Model file for the job. Use its own axes, mm. Face numbers are marked on the shaded views. A direction names the side the tool comes from. Coordinates: 2 decimals unless noted, no trailing zeros. Write each loop counter-clockwise with the first axis right and the second up, starting at its lowest first coordinate (ties: lowest second). Pieces come first, ordered by that corner, then holes.
Q1. Which spindle directions (+Z, -Z, +X, -X, +Y, -Y) get a long thin tool onto all of the face, cutting with end or side? Do the marked faces 1 and 2. Say none if no direction does.
Q2. Band-saw the part on A-A, the plane x = 0. State how many separate pieces and enclosed holes the cut face has, plus the area to 3 significant figures.
Q3. Band-saw the part on B-B, the plane y = -3.4. Write the cut outline in (x, z), plus the area to 3 significant figures.
Q4. Pull direction Z, two halves, no side cores. Call the marked faces 3, 4, 5 and 6: released by +Z, released by -Z, zero draft, split by the parting line, or undercut.
Q5. Pin check, flat tips, straight feed: P1, Ø1.5, axis at y = -4, z = 4, coming from the -X side; P2, Ø2, axis at y = -2, z = -3, coming from the +X side; P3, Ø1, axis at x = 4.5, y = -1, coming from the +Z side; P4, Ø1.5, axis at x = 5, z = 4.5, coming from the +Y side. Stop position of each tip, or through.
Q6. Drill centre lines: probe 1 along Z at (x, y) = (0, -0.95); probe 2 along Z at (x, y) = (0, -3.7); probe 3 along Z at (x, y) = (-1, -1.5). Where is each one in solid material? Low to high.
Autodesk Inventor part; units mm, degrees
ref_plane "YZ Plane" through (0, 0, 0) normal (1, 0, 0) x (0, 1, 0)
ref_plane "XZ Plane" through (0, 0, 0) normal (0, 1, 0) x (-1, 0, 0)
ref_plane "XY Plane" through (0, 0, 0) normal (0, 0, 1) x (1, 0, 0)
sketch "Sketch1" plane through (0, 0, 0) normal (0, 0, 1) x (1, 0, 0)
  line L0 (-12, 0) -> (2, 0) construction
  line L1 (0, -5.4) -> (0, 0.9) construction
  line L2 (-1.5, 0) -> (-10, 0)
  line L3 (-10, 0) -> (-10, -2)
  line L4 (-10, -2) -> (-4.5, -2)
  line L5 (-4.5, -2) -> (-4.5, -4.5)
  line L6 (-4.5, -4.5) -> (-3, -4.5)
  line L7 (-3, -4.5) -> (-3, -2)
  line L8 (-3, -2) -> (-1.5, -2)
  line L9 (-1.5, 0) -> (-1.5, -2)
  point P0 (0, 0)
  dimension "d0" = 1.5
  dimension "d1" = 3
  dimension "d2" = 4.5
  dimension "d3" = 10
  dimension "d4" = 2
  dimension "d5" = 4.5
revolve "Revolution1" add sketch "Sketch1" angle 360 about axis through (0, -10, 0) along (0, 1, 0)
sketch "Sketch2" plane through (0, 0, 0) normal (0, 1, 0) x (1, 0, 0)
  line L0 (-14, 0) -> (14, 0) construction
  line L1 (0, 14) -> (0, -14) construction
  point P0 (0, 0)
  point P1 (0, 7)
  point P2 (0, -7)
  point P3 (-7, 0)
  point P4 (7, 0)
  dimension "d7" = 14
  dimension "d8" = 14
hole "Hole1" at (0, 0, -7) at (0, 0, 7) at (-7, 0, 0) at (7, 0, 0) direction (0, -1, 0) diameter 2.459 depth 8.8
chamfer "Chamfer1" distance 0.25 angle 45 16 edges at (10, 0, 0) (10, -2, 0) (0, 0, -8.2295) (7, 0, -1.2295) (-7, 0, -1.2295) (0, 0, 5.7705) (4.5, -2, 0) (4.5, -4.5, 0) (3, -4.5, 0) (3, -2, 0) (1.5, -2, 0) (1.5, 0, 0) (0, -2, -8.2295) (7, -2, -1.2295) (-7, -2, -1.2295) (0, -2, 5.7705)
properties part number "motortarcsa"
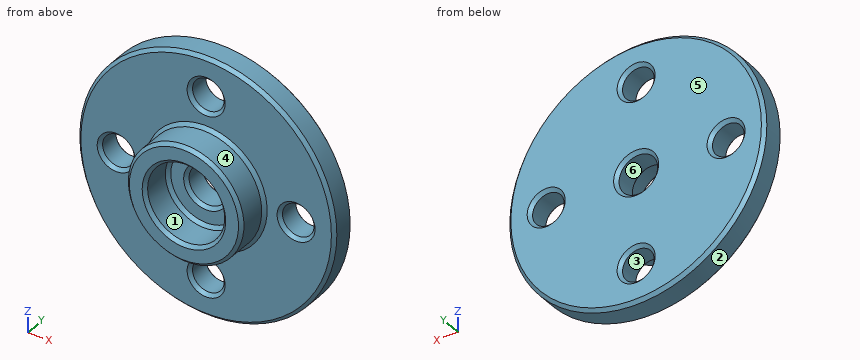
Answer sheet:
1. face 1: -Y
1. face 2: +Y, -Y
2. separate pieces: 4
2. enclosed holes: 0
2. area: 31.2 mm2
3. outline: circle Ø9 at (0, 0); hole circle Ø6 at (0, 0)
3. area: 35.3 mm2
4. face 3: undercut
4. face 4: split by the parting line
4. face 5: zero draft
4. face 6: undercut
5. P1: stops at x = -3.11
5. P2: stops at x = 9.79
5. P3: stops at z = 9.17
5. P4: stops at y = 0
6. probe 1: z = -10 to -8.23, -5.77 to -1.5, 1.5 to 5.77, 8.23 to 10
6. probe 2: z = -4.5 to -3, 3 to 4.5
6. probe 3: z = -9.95 to -7.72, -6.28 to -1.12, 1.12 to 6.28, 7.72 to 9.95
